from build123d import *

# Parameters (mm, degrees)
CROQUIS1_R              = 4
CROQUIS1_R_2            = 30
CROQUIS1_R_3            = 15
SALIENTE_EXTRUIR2_DEPTH = 10


with BuildPart() as part:
    # Croquis1 → Saliente-Extruir2 (new body)
    # profile 1 of 2: a face of its own
    with BuildSketch(Plane.XY):
        with BuildLine():
            ThreePointArc((-80, -14.106158457), (-54.368470232, 13.637354869), (-19.61, 28.42))
            ThreePointArc((-19.61, 28.42), (-13.455358454, 53.846912835), (-14.106158457, 80))
            ThreePointArc((-14.106158457, 80), (13.637354869, 54.368470232), (28.42, 19.61))
            ThreePointArc((28.42, 19.61), (53.846912835, 13.455358454), (80, 14.106158457))
            ThreePointArc((80, 14.106158457), (54.368470232, -13.637354869), (19.61, -28.42))
            ThreePointArc((19.61, -28.42), (13.455358454, -53.846912835), (14.106158457, -80))
            ThreePointArc((14.106158457, -80), (-13.637354869, -54.368470232), (-28.42, -19.61))
            ThreePointArc((-28.42, -19.61), (-53.846912835, -13.455358454), (-80, -14.106158457))
        make_face()
        with Locations((-46.65, -8.22565365)):
            Circle(CROQUIS1_R, mode=Mode.SUBTRACT)
        Circle(CROQUIS1_R_2, mode=Mode.SUBTRACT)
        with Locations((-8.22565365, 46.65)):
            Circle(CROQUIS1_R, mode=Mode.SUBTRACT)
        with Locations((46.65, 8.22565365)):
            Circle(CROQUIS1_R, mode=Mode.SUBTRACT)
        with Locations((8.22565365, -46.65)):
            Circle(CROQUIS1_R, mode=Mode.SUBTRACT)
    # profile 2 of 2: a face of its own
    with BuildSketch(Plane.XY):
        Circle(CROQUIS1_R_2)
        Circle(CROQUIS1_R_3, mode=Mode.SUBTRACT)
    extrude(amount=SALIENTE_EXTRUIR2_DEPTH)


solid = part.part
Geometry check sheet. Reference: the model listing, model coordinates, mm. Round coordinates to 2 decimals unless told otherwise and drop trailing zeros. Order: outer loops, then holes, each group sorted by start corner. A loop starts at its lowest first (then second) coordinate and runs counter-clockwise, first axis right, second up. Notation, with made-up numbers: M -27.75,62 L -12.75,62 A21 ccw -12.75,88 Z; hole C 43.5,86.25 d5. An arc over 180 degrees is marked long. Answer in a Markdown table with one row per item.
(1) Sectioned sample at A-A, the plane y = 46.65. Record the cut outline in (x, z), and give its area (3 significant figures).
Responses:
| item | result |
|---|---|
| outline | M -14.49,0 L -12.23,0 L -12.23,10 L -14.49,10 Z; M -4.23,0 L 18.51,0 L 18.51,10 L -4.23,10 Z |
| area | 250 mm² |
(2) Sectioned sample at D-D, the plane x = 69. Record the cut outline in (y, z).
Responses:
| item | result |
|---|---|
| outline | M -0.75,0 L 12.99,0 L 12.99,10 L -0.75,10 Z |
(3) Draft check along X on faces 1 (the face through (-53.482, -13.495, 4.93)), 2 (the face through (13.495, -53.482, 4.93)), 3 (the face through (-54.8, 13.33, 4.93)). Enter one of: released by +X, released by -X, zero draft, split by the parting line, or undercut.
Responses:
| item | result |
|---|---|
| face 1 | undercut |
| face 2 | released by +X |
| face 3 | released by -X |
(4) Go/stop test with flat-tipped pins: P1, Ø4, axis at y = -32, z = 7.5, coming from the +X side; P2, Ø1.5, axis at y = -48, z = 5.5, coming from the -X side; P3, Ø6.5, axis at x = 8.23, y = -46.65, coming from the +Z side; P4, Ø1, axis at x = 55, z = 3, coming from the -Y side. Record where each tip stops, or that it passes through.
Responses:
| item | result |
|---|---|
| P1 | stops at x = 19.01 |
| P2 | stops at x = -18.17 |
| P3 | passes through |
| P4 | stops at y = -13.54 |
(5) Scan lines: probe 1 along Y at (x, z) = (-46.65, 3.75); probe 2 along X at (y, z) = (6.5, 1); probe 3 along X at (y, z) = (44.5, 6). Record each from-to range of solid material in increasing order. Write a range as from..to.
Responses:
| item | result |
|---|---|
| probe 1 | y = -14.49..-12.23, -4.23..18.51 |
| probe 2 | x = -63.25..-13.52, 13.52..43.04, 50.26..74.96 |
| probe 3 | x = -14.9..-11.6, -4.85..19.68 |
(6) Sectioned sample at B-B, the plane x = 46.65. Record the cut outline in (y, z).
Responses:
| item | result |
|---|---|
| outline | M -18.51,0 L 4.23,0 L 4.23,10 L -18.51,10 Z; M 12.23,0 L 14.49,0 L 14.49,10 L 12.23,10 Z |
(7) Sectioned sample at C-C, the plane z = 1.5. Record the cut outline in (x, y), and give its area (3 significant figures).
Responses:
| item | result |
|---|---|
| outline | M -80,-14.11 A100 cw -28.42,-19.61 A90 ccw 14.11,-80 A100 cw 19.61,-28.42 A90 ccw 80,14.11 A100 cw 28.42,19.61 A90 ccw -14.11,80 A100 cw -19.61,28.42 A90 ccw Z; hole C -46.65,-8.23 d8; hole C 0,0 d30; hole C -8.23,46.65 d8; hole C 8.23,-46.65 d8; hole C 46.65,8.23 d8 |
| area | 7,630 mm² |
